from build123d import *

# Parameters (mm, degrees)
BOSS_EXTRUDE1_DEPTH = 15


with BuildPart() as part:
    # Sketch1 → Boss-Extrude1 (new body)
    with BuildSketch(Plane.XY):
        with BuildLine():
            Line((0, 3), (0, 12))
            ThreePointArc((0, 12), (11, 23), (22, 12))
            Line((22, 12), (22, -13))
            Line((22, -13), (35, -13))
            Line((35, -13), (35, 12))
            ThreePointArc((35, 12), (46, 23), (57, 12))
            Line((57, 12), (57, 3))
            ThreePointArc((57, 3), (59.121320344, -2.121320344), (54, 0))
            Line((54, 0), (54, 12))
            ThreePointArc((54, 12), (46, 20), (38, 12))
            Line((38, 12), (38, -16))
            Line((38, -16), (31.871401461, -16))
            Line((31.871401461, -16), (31.871401461, -28))
            Line((31.871401461, -28), (33.5, -28))
            Line((33.5, -28), (31, -36))
            Line((31, -36), (29.507974066, -36))
            Line((29.507974066, -36), (29.507974066, -20.105540997))
            ThreePointArc((29.507974066, -20.105540997), (29.212255946, -19.395620555), (28.5, -19.10557279))
            ThreePointArc((28.5, -19.10557279), (27.787744054, -19.395620555), (27.492025934, -20.105540997))
            Line((27.492025934, -20.105540997), (27.492025934, -36))
            Line((27.492025934, -36), (26, -36))
            Line((26, -36), (23.5, -28))
            Line((23.5, -28), (25.128598539, -28))
            Line((25.128598539, -28), (25.128598539, -16))
            Line((25.128598539, -16), (19, -16))
            Line((19, -16), (19, 12))
            ThreePointArc((19, 12), (11, 20), (3, 12))
            Line((3, 12), (3, 0))
            ThreePointArc((3, 0), (-2.121320344, -2.121320344), (0, 3))
        make_face()
    extrude(amount=BOSS_EXTRUDE1_DEPTH)


solid = part.part
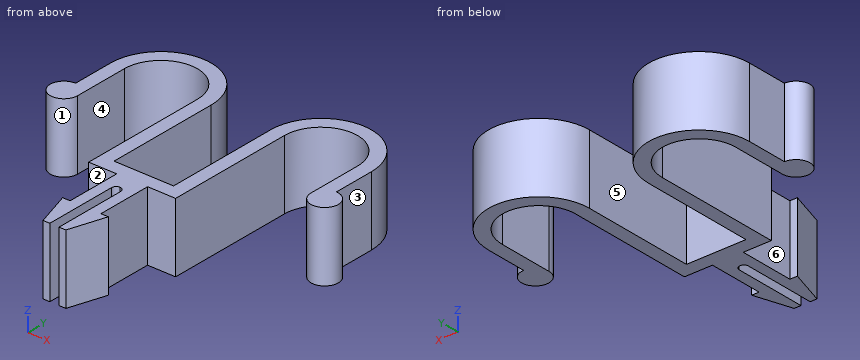
The model under review builds one solid part; all positions refer to its coordinate system, in mm. Face numbers are marked on the shaded views. A direction names the side the tool comes from. Coordinates: 2 decimals unless noted, no trailing zeros. Loops run counter-clockwise (first coordinate to the right, second up) from the corner with the lowest first, then second, coordinate; pieces in that order, holes last.
(1) Draft analysis for pull direction X (two halves, no side actions). For the marked faces 1, 2 and 3, state which applies: +X half, -X half, draft (parallel to the pull), parting line (faces both ways), or undercut.
Determined:
face 1: undercut
face 2: draft
face 3: +X half
(2) Consider section D-D, the plane x = 4. Give the boundary of the cut face in (y, z), plus the area to 3 significant figures.
Determined:
outline: (15.87, 0) - (20.49, 0) - (20.49, 15) - (15.87, 15) - close
area: 69.2 mm2
(3) Consider section A-A, the plane y = -9. Give the boundary of the cut face in (x, z), plus the area to 3 significant figures.
Determined:
outline: (19, 0) - (22, 0) - (22, 15) - (19, 15) - close; (35, 0) - (38, 0) - (38, 15) - (35, 15) - close
area: 90.0 mm2
(4) Wall thickness on L1, parallel to X at y = 8, z = 9; L2, parallel to X at y = -24, z = 3.75; L3, parallel to X at y = 17.5, z = 11: over which ranges is each line inside the solid? List them lowest first.
Determined:
L1: x = 0 to 3, 19 to 22, 35 to 38, 54 to 57
L2: x = 25.13 to 27.49, 29.51 to 31.87
L3: x = 1.47 to 5.19, 16.81 to 20.53, 36.47 to 40.19, 51.81 to 55.53
(5) Insertion check: P1, Ø3.5, axis at y = -21, z = 4, coming from the -X side; P2, Ø6, axis at y = 11, z = 8, coming from the -X side; P3, Ø7.5, axis at y = -1, z = 5.5, coming from the -X side; P4, Ø1.8, axis at x = 24, z = 5.5, coming from the +Y side. Each pin has a flat end and moves straight along its axis. Give the tip position at first contact, or say it passes through.
Determined:
P1: stops at x = 25.13
P2: stops at x = 0
P3: stops at x = -3
P4: stops at y = -13
(6) Tool access review of the marked faces 4, 5 and 6: name each direction out of +Z, -Z, +X, -X, +Y, -Y from which nothing blocks a thin tool from reaching the whole face with its end or side.
Determined:
face 4: +Z, -Z, -Y
face 5: +Z, -Z, +Y
face 6: +Z, -Z, -X
(7) Consider section C-C, the plane x = 11. Give the boundary of the cut face in (y, z), plus the area to 3 significant figures.
Determined:
outline: (20, 0) - (23, 0) - (23, 15) - (20, 15) - close
area: 45.0 mm2
